from build123d import *

# Parameters (mm, degrees)
F0_W     = 59.3514069915
F0_H     = 25.3017321229
F0_W_2   = 2.8294473886
F0_H_2   = 1.1425092816
F0_W_3   = 2.8104633093
F0_H_3   = 1.1491477489
F0_H_4   = 1.1398382485
F0_W_4   = 2.8264205903
F0_H_5   = 1.1500753462
F0_H_6   = 1.1371672153
F2_DEPTH = 2.54
F1_W     = 1.8652155995
F1_H     = 1.7804317176
F1_W_2   = 1.8652137369
F1_W_3   = 1.850374043
F1_H_2   = 1.7718821764
F3_DEPTH = 25.4
F4_DEPTH = 13.716
F5_DEPTH = 17.272


with BuildPart() as f2:
    # F0 (on Front) → F2 (new body)
    with BuildSketch(Plane.XZ):
        with Locations((-45.5565787852, 49.0557551384)):
            Rectangle(F0_W, F0_H)
        with Locations((-67.9233074188, 39.9998538196)):
            Rectangle(F0_W_2, F0_H_2, mode=Mode.SUBTRACT)
        with Locations((-49.0072369576, 39.9998538196)):
            Rectangle(F0_W_3, F0_H_2, mode=Mode.SUBTRACT)
        with Locations((-67.9233074188, 44.3319603801)):
            Rectangle(F0_W_2, F0_H_3, mode=Mode.SUBTRACT)
        with Locations((-67.9233074188, 48.5712159425)):
            Rectangle(F0_W_2, F0_H_4, mode=Mode.SUBTRACT)
        with Locations((-49.0072369576, 44.3319603801)):
            Rectangle(F0_W_3, F0_H_3, mode=Mode.SUBTRACT)
        with Locations((-49.0072369576, 48.5712159425)):
            Rectangle(F0_W_3, F0_H_4, mode=Mode.SUBTRACT)
        with Locations((-29.2699420825, 39.9998538196)):
            Rectangle(F0_W_4, F0_H_2, mode=Mode.SUBTRACT)
        with Locations((-29.2699420825, 44.3319603801)):
            Rectangle(F0_W_4, F0_H_3, mode=Mode.SUBTRACT)
        with Locations((-29.2699420825, 48.5712159425)):
            Rectangle(F0_W_4, F0_H_4, mode=Mode.SUBTRACT)
        with Locations((-67.9233074188, 53.1031731516)):
            Rectangle(F0_W_2, F0_H_5, mode=Mode.SUBTRACT)
        with Locations((-49.0072369576, 53.1031731516)):
            Rectangle(F0_W_3, F0_H_5, mode=Mode.SUBTRACT)
        with Locations((-67.9233074188, 57.1425780654)):
            Rectangle(F0_W_2, F0_H_6, mode=Mode.SUBTRACT)
        with Locations((-49.0072369576, 57.1425780654)):
            Rectangle(F0_W_3, F0_H_6, mode=Mode.SUBTRACT)
        with Locations((-29.2699420825, 53.1031731516)):
            Rectangle(F0_W_4, F0_H_5, mode=Mode.SUBTRACT)
        with Locations((-29.2699420825, 57.1425780654)):
            Rectangle(F0_W_4, F0_H_6, mode=Mode.SUBTRACT)
    extrude(amount=F2_DEPTH)

    # F1 (on Front) → F3 (cut)
    with BuildSketch(Plane.XZ):
        with Locations((-71.5445019305, 59.5189426094)):
            Rectangle(F1_W, F1_H)
        with Locations((-26.1859139428, 59.5189426094)):
            Rectangle(F1_W_2, F1_H)
        with Locations((-71.5519227087, 37.9981175065)):
            Rectangle(F1_W_3, F1_H_2)
        with Locations((-26.1859139428, 37.9981175065)):
            Rectangle(F1_W_2, F1_H_2)
    extrude(amount=F3_DEPTH, mode=Mode.SUBTRACT)

    # F4 (add): a face of the model
    f4_faces = [f2.faces().sort_by_distance(p)[0] for p in [
        (-15.8808752894, -1.27, 49.0557551384),
    ]]
    extrude(f4_faces, amount=F4_DEPTH)

    # F5 (add): a face of the model
    f5_faces = [f2.faces().sort_by_distance(p)[0] for p in [
        (-75.2322822809, -1.27, 49.0557551384),
    ]]
    extrude(f5_faces, amount=F5_DEPTH)


solid = f2.part
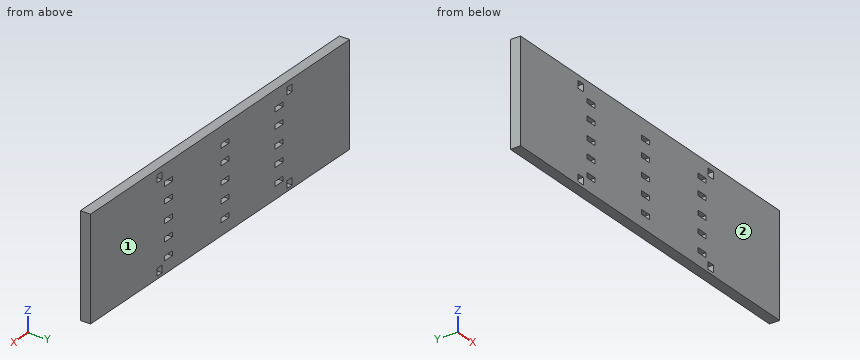
Could you check a few things on this model? Use its own coordinates, in mm. Face numbers are marked on the shaded views. Coordinates: 2 decimals unless noted, no trailing zeros.
Q1. Suppose I cut it at A-A on y = -1.4. Give the number of separate pieces and of enclosed holes in the cut face, and give its area (3 significant figures).
Q2. Please list where these lines run through material, in increasing order: L1, parallel to X at y = -2, z = 49; L2, parallel to Z at x = -29.5, y = -1.7.
Q3. Thinking about a two-plate mould opening in Y: for the marked faces 1 and 2, which applies, released by +Y, released by -Y, zero draft, split by the parting line, or undercut?
Answer:
1. separate pieces: 1
1. enclosed holes: 19
1. area: 2,220 mm2
2. L1: x = -92.5 to -69.34, -66.51 to -50.41, -47.6 to -30.68, -27.86 to -2.16
2. L2: z = 36.4 to 39.43, 40.57 to 43.76, 44.91 to 48, 49.14 to 52.53, 53.68 to 56.57, 57.71 to 61.71
3. face 1: released by +Y
3. face 2: released by -Y
